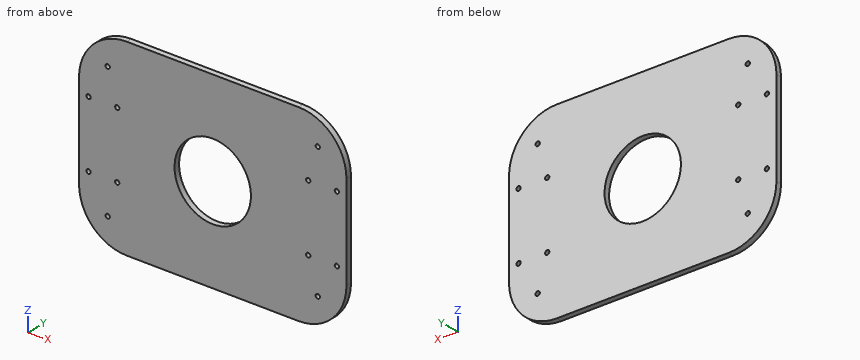
from build123d import *

# Parameters (mm, degrees)
SKETCH_6_W          = 440
SKETCH_6_H          = 200
SKETCH_6_R          = 40
EXTRUDE_2_DEPTH     = 6
SKETCH_7_R          = 2.25
CUT_EXTRUDE_1_DEPTH = 10


with BuildPart() as part:
    # 草图6 → 凸台-拉伸2 (new body)
    with BuildSketch(Plane(origin=(0, 0, 0), x_dir=(1, 0, 0), z_dir=(0, 1, 0))):
        Rectangle(SKETCH_6_W, SKETCH_6_H)
        with Locations(Location((0, 0, 0), (0, 0, 270))):
            Circle(SKETCH_6_R, mode=Mode.SUBTRACT)
    extrude(amount=EXTRUDE_2_DEPTH)

    # 草图7 → 切除-拉伸1 (cut)
    with BuildSketch(Plane(origin=(0, 6, 0), x_dir=(1, 0, 0), z_dir=(0, 1, 0))):
        with BuildLine():
            Line((-140, -50), (-140, 50))
            ThreePointArc((-140, 50), (-125.355339059, 85.355339059), (-90, 100))
            Line((-90, 100), (-220, 100))
            Line((-220, 100), (-220, -100))
            Line((-220, -100), (-90, -100))
            ThreePointArc((-90, -100), (-125.355339059, -85.355339059), (-140, -50))
        make_face()
        with BuildLine():
            Line((220, 100), (90, 100))
            ThreePointArc((90, 100), (125.355339059, 85.355339059), (140, 50))
            Line((140, 50), (140, -50))
            ThreePointArc((140, -50), (125.355339059, -85.355339059), (90, -100))
            Line((90, -100), (220, -100))
            Line((220, -100), (220, 100))
        make_face()
        with Locations(Location((-130, 35, 0), (0, 0, 270))):
            Circle(SKETCH_7_R)
        with Locations(Location((-100, 35, 0), (0, 0, 270))):
            Circle(SKETCH_7_R)
        with Locations(Location((-110, 70, 0), (0, 0, 270))):
            Circle(SKETCH_7_R)
        with Locations(Location((110, 70, 0), (0, 0, 270))):
            Circle(SKETCH_7_R)
        with Locations(Location((100, 35, 0), (0, 0, 270))):
            Circle(SKETCH_7_R)
        with Locations(Location((130, 35, 0), (0, 0, 270))):
            Circle(SKETCH_7_R)
        with Locations(Location((130, -35, 0), (0, 0, 270))):
            Circle(SKETCH_7_R)
        with Locations(Location((100, -35, 0), (0, 0, 270))):
            Circle(SKETCH_7_R)
        with Locations(Location((110, -70, 0), (0, 0, 270))):
            Circle(SKETCH_7_R)
        with Locations(Location((-110, -70, 0), (0, 0, 270))):
            Circle(SKETCH_7_R)
        with Locations(Location((-100, -35, 0), (0, 0, 270))):
            Circle(SKETCH_7_R)
        with Locations(Location((-130, -35, 0), (0, 0, 270))):
            Circle(SKETCH_7_R)
    extrude(amount=-CUT_EXTRUDE_1_DEPTH, mode=Mode.SUBTRACT)


solid = part.part
The listing builds one solid part. Answer for the finished solid, in the listing's coordinates (mm). Give positions to 0.01 mm unless a question says otherwise; leave off trailing zeros. Write each loop counter-clockwise with the first axis right and the second up, starting at its lowest first coordinate (ties: lowest second). Pieces come first, ordered by that corner, then holes.
1) Section B-B (y = 1.1) is taken. Count the separate pieces of the cut face and the enclosed holes in it, and give its area (3 significant figures).
2) Find the intervals of material crossed by L1, parallel to X at y = 4.8, z = 35; L2, parallel to X at y = 4.1, z = 70; L3, parallel to X at y = 4.4, z = -16, in increasing order.
3) Given P1, Ø3.5, axis at x = 100, z = 35, coming from the -Y side, flat-ended and moving along its own axis, determine where the tip first touches the part or whether it passes through.
4) Section A-A (x = -8.5) is taken. Write down the section's boundary in (y, z).
5) Section C-C (z = -20.5) is taken. Write down the section's boundary in (x, y), and give its area (3 significant figures).
Response:
1. separate pieces: 1
1. enclosed holes: 13
1. area: 48,600 mm2
2. L1: x = -140 to -132.25, -127.75 to -102.25, -97.75 to -19.36, 19.36 to 97.75, 102.25 to 127.75, 132.25 to 140
2. L2: x = -135.83 to -112.25, -107.75 to 107.75, 112.25 to 135.83
2. L3: x = -140 to -36.66, 36.66 to 140
3. P1: passes through
4. outline: (0, -100) - (6, -100) - (6, -39.09) - (0, -39.09) - close; (0, 39.09) - (6, 39.09) - (6, 100) - (0, 100) - close
5. outline: (-140, 0) - (-34.35, 0) - (-34.35, 6) - (-140, 6) - close; (34.35, 0) - (140, 0) - (140, 6) - (34.35, 6) - close
5. area: 1,270 mm2
